The model under review builds one solid part; all positions refer to its coordinate system, in mm. Round coordinates to 2 decimals unless told otherwise and drop trailing zeros. Answer as a JSON object with one key per item and string values. Group by question number.
Item 1: Consider section A-A (y = 219). State how many separate pieces and enclosed holes the cut face has, and give its area (3 significant figures).
Item 2: To check wall thickness, follow line 1 (Z direction, x = 1.6, y = 112.5); line 2 (Y direction, x = 0.4, z = -13); line 3 (Y direction, x = 0.6, z = -102). State the ranges of each line that lie inside material, in increasing order.
Item 3: Insertion check: P1, Ø1, axis at y = 226, z = -138, coming from the +X side. The pin has a flat end and moves straight along its axis. Give the tip position at first contact, or say it passes through.
```python
from build123d import *

# Parameters (mm, degrees)
SKETCH_1_W             = 188
SKETCH_1_H             = 260.5
BASE_DEPTH             = 1.8
SKETCH_3_R             = 1.525
SKETCH_3_R_2           = 2
SKETCH_3_R_3           = 1.5
SKETCH_3_W             = 120
SKETCH_3_H             = 12
PCIE_DEPTH             = 1.8
CUT_EXTRUDE_2024_REACH = 323.259
SKETCH_5_W             = 18
SKETCH_5_H             = 22
CUT_EXTRUDE_3211_REACH = 323.259
SKETCH_4_R             = 2
THER_DEPTH             = 1.8
FILLET_1_R             = 1.5
FILLET_2_R             = 0.8


with BuildPart() as part:
    # 草图1 → base (new body)
    with BuildSketch(Plane(origin=(0, 0, 0), x_dir=(0, 0, -1), z_dir=(1, 0, 0))):
        with Locations((94, 130.25)):
            Rectangle(SKETCH_1_W, SKETCH_1_H)
    extrude(amount=BASE_DEPTH)

    # 草图3 → pcie (cut)
    with BuildSketch(Plane(origin=(1.8, 0, 0), x_dir=(0, 0, -1), z_dir=(1, 0, 0))):
        with Locations((13.5, 249.8)):
            Circle(SKETCH_3_R)
        with Locations((174.5, 249.8)):
            Circle(SKETCH_3_R)
        with Locations((156.45, 150.5)):
            Circle(SKETCH_3_R_2)
        with Locations((41, 130.5)):
            Circle(SKETCH_3_R_3)
        with Locations((148.45, 130.5)):
            Circle(SKETCH_3_R_3)
        with Locations((27, 150.5)):
            Circle(SKETCH_3_R_2)
        with Locations((26.5, 114.7)):
            Circle(SKETCH_3_R_2)
        with Locations((142.45, 114.7)):
            Circle(SKETCH_3_R_2)
        with Locations((27, 174.5)):
            Circle(SKETCH_3_R_2)
        with Locations((156.45, 174.5)):
            Circle(SKETCH_3_R_2)
        with Locations((94.725, 137.5)):
            Circle(SKETCH_3_R_2)
        with Locations((94.725, 123.5)):
            Circle(SKETCH_3_R_2)
        with Locations((94.725, 95.8)):
            Rectangle(SKETCH_3_W, SKETCH_3_H)
        with BuildLine():
            Line((15.025, 10.9), (15.025, 9.9))
            ThreePointArc((15.025, 9.9), (13.5, 8.375), (11.975, 9.9))
            Line((11.975, 9.9), (11.975, 10.9))
            ThreePointArc((11.975, 10.9), (13.5, 12.425), (15.025, 10.9))
        make_face()
        with BuildLine():
            Line((176.025, 10.9), (176.025, 9.9))
            ThreePointArc((176.025, 9.9), (174.5, 8.375), (172.975, 9.9))
            Line((172.975, 9.9), (172.975, 10.9))
            ThreePointArc((172.975, 10.9), (174.5, 12.425), (176.025, 10.9))
        make_face()
    extrude(amount=-PCIE_DEPTH, mode=Mode.SUBTRACT)

    # 草图5 → Cut-Extrude 2024 (cut, up to next)
    with BuildSketch(Plane(origin=(1.8, 0, 0), x_dir=(0, 0, -1), z_dir=(1, 0, 0)), mode=Mode.PRIVATE) as cut_extrude_2024_sk1:
        with Locations((168.6, 118.3)):
            Rectangle(SKETCH_5_W, SKETCH_5_H)
    cut_extrude_2024_tool1 = extrude(cut_extrude_2024_sk1.sketch, amount=-CUT_EXTRUDE_2024_REACH, mode=Mode.PRIVATE) & part.part
    add(cut_extrude_2024_tool1.solids().sort_by_distance((1.8, 118.3, -168.6))[0], mode=Mode.SUBTRACT)

    # 草图4 → Cut-Extrude 3211 (cut, up to next)
    with BuildSketch(Plane(origin=(1.8, 0, 0), x_dir=(0, 0, -1), z_dir=(1, 0, 0)), mode=Mode.PRIVATE) as cut_extrude_3211_sk1:
        with Locations((114.5, 83.8)):
            Circle(SKETCH_4_R)
    cut_extrude_3211_tool1 = extrude(cut_extrude_3211_sk1.sketch, amount=-CUT_EXTRUDE_3211_REACH, mode=Mode.PRIVATE) & part.part
    # 草图4 → Cut-Extrude 3211 (cut, up to next)
    with BuildSketch(Plane(origin=(1.8, 0, 0), x_dir=(0, 0, -1), z_dir=(1, 0, 0)), mode=Mode.PRIVATE) as cut_extrude_3211_sk2:
        with Locations((176, 83.8)):
            Circle(SKETCH_4_R)
    cut_extrude_3211_tool2 = extrude(cut_extrude_3211_sk2.sketch, amount=-CUT_EXTRUDE_3211_REACH, mode=Mode.PRIVATE) & part.part
    # 草图4 → Cut-Extrude 3211 (cut, up to next)
    with BuildSketch(Plane(origin=(1.8, 0, 0), x_dir=(0, 0, -1), z_dir=(1, 0, 0)), mode=Mode.PRIVATE) as cut_extrude_3211_sk3:
        with Locations((176, 22.3)):
            Circle(SKETCH_4_R)
    cut_extrude_3211_tool3 = extrude(cut_extrude_3211_sk3.sketch, amount=-CUT_EXTRUDE_3211_REACH, mode=Mode.PRIVATE) & part.part
    # 草图4 → Cut-Extrude 3211 (cut, up to next)
    with BuildSketch(Plane(origin=(1.8, 0, 0), x_dir=(0, 0, -1), z_dir=(1, 0, 0)), mode=Mode.PRIVATE) as cut_extrude_3211_sk4:
        with Locations((114.5, 22.3)):
            Circle(SKETCH_4_R)
    cut_extrude_3211_tool4 = extrude(cut_extrude_3211_sk4.sketch, amount=-CUT_EXTRUDE_3211_REACH, mode=Mode.PRIVATE) & part.part
    add(cut_extrude_3211_tool1.solids().sort_by_distance((1.8, 83.8, -114.5))[0], mode=Mode.SUBTRACT)
    add(cut_extrude_3211_tool2.solids().sort_by_distance((1.8, 83.8, -176))[0], mode=Mode.SUBTRACT)
    add(cut_extrude_3211_tool3.solids().sort_by_distance((1.8, 22.3, -176))[0], mode=Mode.SUBTRACT)
    add(cut_extrude_3211_tool4.solids().sort_by_distance((1.8, 22.3, -114.5))[0], mode=Mode.SUBTRACT)

    # 草图2 → ther (cut)
    with BuildSketch(Plane(origin=(1.8, 0, 0), x_dir=(0, 0, -1), z_dir=(1, 0, 0))):
        with BuildLine():
            Line((58.4375, 235.5), (58.4375, 150.5))
            ThreePointArc((58.4375, 150.5), (55.1875, 147.25), (51.9375, 150.5))
            Line((51.9375, 150.5), (51.9375, 235.5))
            ThreePointArc((51.9375, 235.5), (55.1875, 238.75), (58.4375, 235.5))
        make_face()
        with BuildLine():
            Line((70.625, 235.5), (70.625, 150.5))
            ThreePointArc((70.625, 150.5), (67.375, 147.25), (64.125, 150.5))
            Line((64.125, 150.5), (64.125, 235.5))
            ThreePointArc((64.125, 235.5), (67.375, 238.75), (70.625, 235.5))
        make_face()
        with BuildLine():
            Line((82.8125, 235.5), (82.8125, 150.5))
            ThreePointArc((82.8125, 150.5), (79.5625, 147.25), (76.3125, 150.5))
            Line((76.3125, 150.5), (76.3125, 235.5))
            ThreePointArc((76.3125, 235.5), (79.5625, 238.75), (82.8125, 235.5))
        make_face()
        with BuildLine():
            Line((95, 235.5), (95, 150.5))
            ThreePointArc((95, 150.5), (91.75, 147.25), (88.5, 150.5))
            Line((88.5, 150.5), (88.5, 235.5))
            ThreePointArc((88.5, 235.5), (91.75, 238.75), (95, 235.5))
        make_face()
        with BuildLine():
            Line((107.1875, 235.5), (107.1875, 150.5))
            ThreePointArc((107.1875, 150.5), (103.9375, 147.25), (100.6875, 150.5))
            Line((100.6875, 150.5), (100.6875, 235.5))
            ThreePointArc((100.6875, 235.5), (103.9375, 238.75), (107.1875, 235.5))
        make_face()
        with BuildLine():
            Line((119.375, 235.5), (119.375, 150.5))
            ThreePointArc((119.375, 150.5), (116.125, 147.25), (112.875, 150.5))
            Line((112.875, 150.5), (112.875, 235.5))
            ThreePointArc((112.875, 235.5), (116.125, 238.75), (119.375, 235.5))
        make_face()
        with BuildLine():
            Line((131.5625, 235.5), (131.5625, 150.5))
            ThreePointArc((131.5625, 150.5), (128.3125, 147.25), (125.0625, 150.5))
            Line((125.0625, 150.5), (125.0625, 235.5))
            ThreePointArc((125.0625, 235.5), (128.3125, 238.75), (131.5625, 235.5))
        make_face()
        with BuildLine():
            Line((143.75, 235.5), (143.75, 150.5))
            ThreePointArc((143.75, 150.5), (140.5, 147.25), (137.25, 150.5))
            Line((137.25, 150.5), (137.25, 235.5))
            ThreePointArc((137.25, 235.5), (140.5, 238.75), (143.75, 235.5))
        make_face()
        with BuildLine():
            Line((121.5, 83.8), (169, 83.8))
            ThreePointArc((169, 83.8), (172.5, 80.3), (169, 76.8))
            Line((169, 76.8), (121.5, 76.8))
            ThreePointArc((121.5, 76.8), (118, 80.3), (121.5, 83.8))
        make_face()
        with BuildLine():
            Line((121.5, 29.3), (169, 29.3))
            ThreePointArc((169, 29.3), (172.5, 25.8), (169, 22.3))
            Line((169, 22.3), (121.5, 22.3))
            ThreePointArc((121.5, 22.3), (118, 25.8), (121.5, 29.3))
        make_face()
        with BuildLine():
            Line((114.5, 72.9), (176, 72.9))
            ThreePointArc((176, 72.9), (179.5, 69.4), (176, 65.9))
            Line((176, 65.9), (114.5, 65.9))
            ThreePointArc((114.5, 65.9), (111, 69.4), (114.5, 72.9))
        make_face()
        with BuildLine():
            Line((114.5, 62), (176, 62))
            ThreePointArc((176, 62), (179.5, 58.5), (176, 55))
            Line((176, 55), (114.5, 55))
            ThreePointArc((114.5, 55), (111, 58.5), (114.5, 62))
        make_face()
        with BuildLine():
            Line((114.5, 51.1), (176, 51.1))
            ThreePointArc((176, 51.1), (179.5, 47.6), (176, 44.1))
            Line((176, 44.1), (114.5, 44.1))
            ThreePointArc((114.5, 44.1), (111, 47.6), (114.5, 51.1))
        make_face()
        with BuildLine():
            Line((114.5, 40.2), (176, 40.2))
            ThreePointArc((176, 40.2), (179.5, 36.7), (176, 33.2))
            Line((176, 33.2), (114.5, 33.2))
            ThreePointArc((114.5, 33.2), (111, 36.7), (114.5, 40.2))
        make_face()
    extrude(amount=-THER_DEPTH, mode=Mode.SUBTRACT)

    # 圆角1
    fillet_1_edges = [part.edges().sort_by_distance(p)[0] for p in [
        (0.9, 260.5, 0),
        (0.9, 260.5, -188),
        (0.9, 0, -188),
        (0.9, 0, 0),
    ]]
    fillet(fillet_1_edges, radius=FILLET_1_R)

    # 圆角2
    fillet_2_edges = [part.edges().sort_by_distance(p)[0] for p in [
        (0.9, 107.3, -159.6),
        (0.9, 129.3, -159.6),
        (0.9, 129.3, -177.6),
        (0.9, 107.3, -177.6),
        (0.9, 89.8, -154.725),
        (0.9, 101.8, -154.725),
        (0.9, 101.8, -34.725),
        (0.9, 89.8, -34.725),
    ]]
    fillet(fillet_2_edges, radius=FILLET_2_R)


solid = part.part
```
Geometry results:
{
 "1": {"separate pieces": "9", "enclosed holes": "0", "area": "245 mm^2"},
 "2": {"line 1": "z = -188 to -177.6, -159.6 to 0", "line 2": "y = 0 to 8.46, 12.34 to 248.36, 251.24 to 260.5", "line 3": "y = 0 to 89.8, 101.8 to 147.89, 238.11 to 260.5"},
 "3": {"P1": "passes through"}
}
